from build123d import *

# Parameters (mm, degrees)
SKETCH1_R           = 3.1115
BOSS_EXTRUDE1_DEPTH = 71.12
CUT_EXTRUDE1_DEPTH  = 12
SKETCH3_R           = 1
CUT_EXTRUDE2_DEPTH  = 2.54


with BuildPart() as part:
    # Sketch1 → Boss-Extrude1 (new body)
    with BuildSketch(Plane(origin=(0, 0, 0), x_dir=(0, 0, -1), z_dir=(1, 0, 0))):
        Circle(SKETCH1_R)
    extrude(amount=BOSS_EXTRUDE1_DEPTH)

    # Sketch2 → Cut-Extrude1 (cut)
    with BuildSketch(Plane.ZY):
        with BuildLine():
            Line((-1.151593115, 1.651), (1.151593115, 1.651))
            ThreePointArc((1.151593115, 1.651), (0, -2.01295), (-1.151593115, 1.651))
        make_face()
    extrude(amount=-CUT_EXTRUDE1_DEPTH, mode=Mode.SUBTRACT)

    # Sketch3 → Cut-Extrude2 (cut)
    with BuildSketch(Plane.XZ.offset(-1.651)):
        with Locations((6.288563634, 0)):
            Circle(SKETCH3_R)
    extrude(amount=-CUT_EXTRUDE2_DEPTH, mode=Mode.SUBTRACT)


solid = part.part
Here's how the part is built. I have some questions about the finished solid (model axes, mm). A direction names the side the tool comes from. Give positions to 0.01 mm unless a question says otherwise; leave off trailing zeros. Order: outer loops, then holes, each group sorted by start corner. A loop starts at its lowest first (then second) coordinate and runs counter-clockwise, first axis right, second up. Notation, with made-up numbers: (-38, 36.25) -> (-7, 36.25) arc R13 cw to (-7, 61.25) -> close; hole circle Ø1 at (32, -1.5). An arc over 180 degrees is marked (long way). One line per item, written item: value. Start each with the question number.
1. Imagine slicing it at A-A, the plane z = 0. List the corners of the cut face in (x, y) for me, plus the area to 3 significant figures.
2. Imagine slicing it at B-B, the plane y = 0. List the corners of the cut face in (x, z) for me.
3. I need wall thicknesses on probe 1 along X at (y, z) = (2.5, 0); probe 2 along Y at (x, z) = (8, 0); probe 3 along X at (y, z) = (-1, 1.5). Which ranges of each line are inside material? Lowest first, please. Write a range as from..to.
4. We'd pull the mould along Y, two halves only. Please class faces 1 (the face through (0, -1, -2)), 2 (the face through (35.06, -3.04, 0.67)), 3 (the face through (5, 1.651, 0)): released by +Y, released by -Y, zero draft, split by the parting line, or undercut.
5. Will these pins go through, and if not, where does the flat tip stop? pin 1 Ø2.5 at (y, z) = (0, 0) entering from -X; pin 2 Ø3 at (x, z) = (45, 0.5) entering from -Y; pin 3 Ø1.5 at (x, z) = (63.5, 1.5) entering from -Y.
6. Imagine slicing it at C-C, the plane x = 32.5. List the corners of the cut face in (y, z) for me.
7. For faces 4 (the face through (5.29, 2.37, 0.04)), 5 (the face through (5.92, -2.01, 0.07)), 6 (the face through (71.12, 0, 0)), which set-ups out of +Z, -Z, +X, -X, +Y, -Y let a thin tool reach every point of the face, with its end or its side?
Values follow:
1. outline: (0, -3.11) -> (71.12, -3.11) -> (71.12, 3.11) -> (7.29, 3.11) -> (7.29, 1.65) -> (12, 1.65) -> (12, -2.01) -> (0, -2.01) -> close; (0, 1.65) -> (5.29, 1.65) -> (5.29, 3.11) -> (0, 3.11) -> close
1. area: 396 mm2
2. outline: (0, -3.11) -> (71.12, -3.11) -> (71.12, 3.11) -> (0, 3.11) -> (0, 2.01) -> (12, 2.01) -> (12, -2.01) -> (0, -2.01) -> close
3. probe 1: x = 0..5.29, 7.29..71.12
3. probe 2: y = -3.11..-2.01, 1.65..3.11
3. probe 3: x = 12..71.12
4. face 1: zero draft
4. face 2: split by the parting line
4. face 3: undercut
5. pin 1: stops at x = 12
5. pin 2: stops at y = -3.11
5. pin 3: stops at y = -3.02
6. outline: circle Ø6.22 at (0, 0)
7. face 4: +Y
7. face 5: -X
7. face 6: +Z, -Z, +X, +Y, -Y
